Source: CAD feature listing. Evaluate the final solid. Frame: model axes, mm. Face numbers are marked on the shaded views. A direction names the side the tool comes from. Round coordinates to 2 decimals unless told otherwise and drop trailing zeros. Write each loop counter-clockwise with the first axis right and the second up, starting at its lowest first coordinate (ties: lowest second). Pieces come first, ordered by that corner, then holes. Notation, with made-up numbers: M 61.5,-14.5 L 104.5,-14.5 A13 cw 104.5,1.5 Z; hole C 34,45 d2. An arc over 180 degrees is marked long. Use a Markdown table: item, result.
Autodesk Inventor part; units mm, degrees
ref_plane "YZ Plane" through (0, 0, 0) normal (1, 0, 0) x (0, 1, 0)
ref_plane "XZ Plane" through (0, 0, 0) normal (0, 1, 0) x (-1, 0, 0)
ref_plane "XY Plane" through (0, 0, 0) normal (0, 0, 1) x (1, 0, 0)
sketch "Sketch1" plane through (0, 0, 0) normal (0, 1, 0) x (-1, 0, 0)
  line L0 (0, 0) -> (25.4, 0)
  line L1 (25.4, 0) -> (25.4, 25.4)
  line L2 (25.4, 25.4) -> (0, 25.4)
  line L3 (0, 25.4) -> (0, 0)
  line L4 (22.225, 22.225) -> (22.225, 3.175)
  line L5 (22.225, 3.175) -> (3.175, 3.175)
  line L6 (3.175, 3.175) -> (3.175, 22.225)
  line L7 (3.175, 22.225) -> (22.225, 22.225)
  dimension "d0" = 25.4
  dimension "d1" = 25.4
  dimension "d2" = 3.175
extrude "Extrusion1" add sketch "Sketch1" along normal blind 203.2
sketch "Sketch2" plane through (-25.4, 0, 25.4) normal (0, 0, 1) x (1, 0, 0)
  circle A0 centre (12.7, 12.7) radius 2.5797
  circle A1 centre (12.7, 60.325) radius 2.5797
  line L0 (25.4, 0) -> (25.4, 203.2)
  line L1 (0, 0) -> (25.4, 0)
  circle A2 centre (12.7, 36.5125) radius 9.525
  circle A3 centre (12.7, 190.5) radius 3.3734
  line L2 (0, 0) -> (0, 203.2)
  line L3 (25.4, 203.2) -> (0, 203.2)
  dimension "d5" = 5.1594
  dimension "d6" = 5.1594
  dimension "d7" = 47.625
  dimension "d8" = 12.7
  dimension "d9" = 12.7
  dimension "d10" = 12.7
  dimension "d13" = 19.05
  dimension "d14" = 23.8125
  dimension "d15" = 12.7
  dimension "d16" = 6.7469
  dimension "d17" = 12.7
  dimension "d18" = 12.7
extrude "Extrusion2" cut sketch "Sketch2" against normal blind 25.4 contours A0 | A1 | A2 | A3
properties part number "arm replacement"
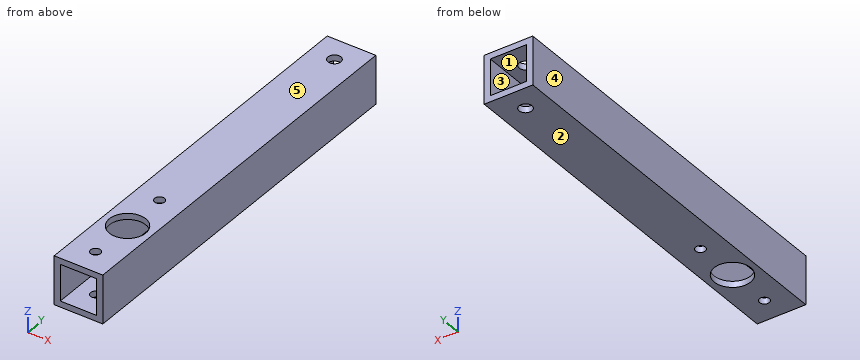
Q1. Section B-B on z = 11.25. Return loops of the section in (x, y) (3 decimals).
Results are:
| item | result |
|---|---|
| outline | M -25.4,0 L -22.225,0 L -22.225,203.2 L -25.4,203.2 Z; M -3.175,0 L 0,0 L 0,203.2 L -3.175,203.2 Z |
Q2. First-contact query: pin 1 Ø3 at (x, y) = (-12.7, 60.325) entering from -Z. Flat tip, straight axial feed; report the tip coordinate or a pass-through.
Results are:
| item | result |
|---|---|
| pin 1 | through |
Q3. Mould query, pull axis Z, two halves, no side actions, for the marked faces 3, 4 and 5. Classes: +Z half, -Z half, draft (parallel to the pull), parting line (faces both ways), or undercut.
Results are:
| item | result |
|---|---|
| face 3 | undercut |
| face 4 | draft |
| face 5 | +Z half |
Q4. Reachability of the marked faces 1 and 2 from +Z, -Z, +X, -X, +Y, -Y: full face, straight path, thin tool, end or side. Return the list, or none.
Results are:
| item | result |
|---|---|
| face 1 | +Y, -Y |
| face 2 | -Z, +X, -X, +Y, -Y |
Q5. Section C-C on y = 143. Return loops of the section in (x, z) (3 decimals).
Results are:
| item | result |
|---|---|
| outline | M -25.4,0 L 0,0 L 0,25.4 L -25.4,25.4 Z; hole M -22.225,3.175 L -3.175,3.175 L -3.175,22.225 L -22.225,22.225 Z |
Q6. Section A-A on y = 190.5. Return loops of the section in (x, z) (3 decimals), plus the area to 3 significant figures.
Results are:
| item | result |
|---|---|
| outline | M -25.4,0 L -16.073,0 L -16.073,3.175 L -22.225,3.175 L -22.225,22.225 L -16.073,22.225 L -16.073,25.4 L -25.4,25.4 Z; M -9.327,0 L 0,0 L 0,25.4 L -9.327,25.4 L -9.327,22.225 L -3.175,22.225 L -3.175,3.175 L -9.327,3.175 Z |
| area | 239 mm^2 |
Q7. Section D-D on x = -12.7. Give the number of separate pieces and of enclosed holes in the cut face, plus the area to 3 significant figures.
Results are:
| item | result |
|---|---|
| separate pieces | 10 |
| enclosed holes | 0 |
| area | 1,060 mm^2 |
Q8. Line query: L1, parallel to Y at x = -12.7, z = 23.8; L2, parallel to Z at x = -3.75, y = 70 (3 decimals); L3, parallel to X at y = 58, z = 5 (3 decimals). Output: solid intervals per line, ascending.
Results are:
| item | result |
|---|---|
| L1 | 0 to 10.12, 15.28 to 26.99, 46.04 to 57.75, 62.9 to 187.13, 193.87 to 203.2 |
| L2 | 0 to 3.175, 22.225 to 25.4 |
| L3 | -25.4 to -22.225, -3.175 to 0 |
